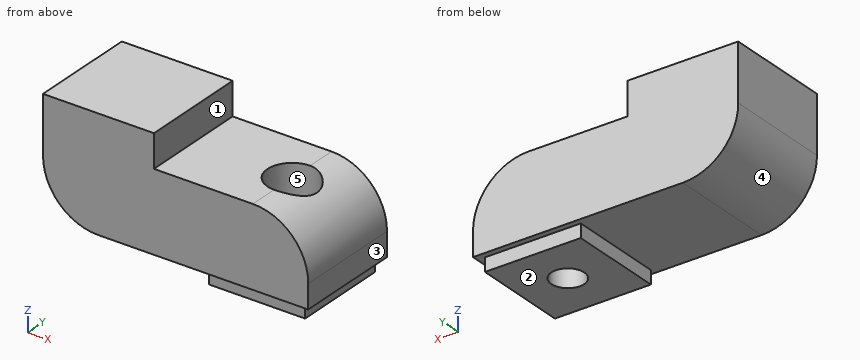
```python
from build123d import *

# Parameters (mm, degrees)
F0_W           = 88.5
F0_H           = 26.5
F1_DEPTH       = 18
F2_W           = 37
F2_H           = 36
F3_DEPTH       = 11
F4_R           = 18.5
F6_W           = 32
F6_H           = 32
F7_DEPTH       = 4.5
F8_D           = 11
F8_CBORE_D     = 16.5
F8_CBORE_DEPTH = 12


with BuildPart() as f1:
    # F0 (on Front) → F1 (new body, symmetric)
    with BuildSketch(Plane.XZ):
        Rectangle(F0_W, F0_H)
    extrude(amount=F1_DEPTH, both=True)

    # F2 (on face) → F3 (join)
    with BuildSketch(Plane.XY.offset(13.25)):
        with Locations((-25.75, 0)):
            Rectangle(F2_W, F2_H)
    extrude(amount=F3_DEPTH)

    # F4
    f4_edges = [f1.edges().sort_by_distance(p)[0] for p in [
        (44.25, 0, 13.25),
        (-44.25, 0, -13.25),
    ]]
    fillet(f4_edges, radius=F4_R)

    # F6 (on face) → F7 (join)
    with BuildSketch(Plane(origin=(0, 0, -13.25), x_dir=(1, 0, 0), z_dir=(0, 0, -1))):
        with Locations((25.75, 0)):
            Rectangle(F6_W, F6_H)
    extrude(amount=F7_DEPTH)

    # F8 (through all)
    with Locations(Plane.XY.offset(13.25)):
        with Locations((25.75, 0)):
            CounterBoreHole(F8_D / 2, F8_CBORE_D / 2, F8_CBORE_DEPTH)


solid = f1.part
```
Source: CAD feature listing. Evaluate the final solid. Frame: model axes, mm. Face numbers are marked on the shaded views. A direction names the side the tool comes from. Round coordinates to 2 decimals unless told otherwise and drop trailing zeros. Loops run counter-clockwise (first coordinate to the right, second up) from the corner with the lowest first, then second, coordinate; pieces in that order, holes last.
1. Mould query, pull axis X, two halves, no side actions, for the marked faces 3, 4 and 5. Classes: released by +X, released by -X, zero draft, split by the parting line, or undercut.
2. Section query D-D on z = -11.5. Output: boundary loops of the cut face in (x, y), and give its area (3 significant figures).
3. Ray query, L1, parallel to Y at x = 25.5, z = 8; L2, parallel to Z at x = 19, y = -7.5; L3, parallel to X at y = 12, z = 13.5. Return the intervals inside material, ascending.
4. Section query B-B on x = 11. Output: boundary loops of the cut face in (y, z).
5. Section query A-A on y = 0. Output: boundary loops of the cut face in (x, z), and give its area (3 significant figures).
6. Access query for the marked faces 1 and 2. Directions: +Z, -Z, +X, -X, +Y, -Y. A direction counts if a zero-diameter tool reaches every point of the face in a straight line with its end or side. Return the directions, or none.
7. Contact query for flat-ended pins moving along their axis: pin 1 (3.5 mm diameter, centred on x = 23.5, z = -16, fed in from -Y); pin 2 (2 mm diameter, centred on y = 5.5, z = -16, fed in from -X); pin 3 (12 mm diameter, centred on y = 8.5, z = 9, fed in from +X). Output: stop coordinate, or through.
8. Section query C-C on y = 13.5. Output: boundary loops of the cut face in (x, z), and give its area (3 significant figures).
Answers below:
1. face 3: released by +X
1. face 4: released by -X
1. face 5: undercut
2. outline: (-33.6, -18) - (44.25, -18) - (44.25, 18) - (-33.6, 18) - close; hole circle Ø11 at (25.75, 0)
2. area: 2,710 mm2
3. L1: y = -18 to -8.25, 8.25 to 18
3. L2: z = -17.75 to 13.25
3. L3: x = -44.25 to -7.25
4. outline: (-18, -13.25) - (-16, -13.25) - (-16, -17.75) - (16, -17.75) - (16, -13.25) - (18, -13.25) - (18, 13.25) - (-18, 13.25) - close
5. outline: (-44.25, 5.25) arc R18.5 ccw to (-25.75, -13.25) - (9.75, -13.25) - (9.75, -17.75) - (20.25, -17.75) - (20.25, 1.25) - (17.5, 1.25) - (17.5, 13.25) - (-7.25, 13.25) - (-7.25, 24.25) - (-44.25, 24.25) - close; (31.25, -17.75) - (41.75, -17.75) - (41.75, -13.25) - (44.25, -13.25) - (44.25, -5.25) arc R18.5 ccw to (34, 11.31) - (34, 1.25) - (31.25, 1.25) - close
5. area: 2,350 mm2
6. face 1: +Z, +X, +Y, -Y
6. face 2: -Z, +X, -X, +Y, -Y
7. pin 1: stops at y = -16
7. pin 2: stops at x = 9.75
7. pin 3: stops at x = 42.31
8. outline: (-44.25, 5.25) arc R18.5 ccw to (-25.75, -13.25) - (9.75, -13.25) - (9.75, -17.75) - (41.75, -17.75) - (41.75, -13.25) - (44.25, -13.25) - (44.25, -5.25) arc R18.5 ccw to (25.75, 13.25) - (-7.25, 13.25) - (-7.25, 24.25) - (-44.25, 24.25) - close
8. area: 2,750 mm2
